from build123d import *

# Parameters (mm, degrees)
CROQUIS2_W                 = 25
CROQUIS2_H                 = 50
SALIENTE_EXTRUIR2_DEPTH    = 20
CROQUIS19_W                = 25
CROQUIS19_H                = 20
SALIENTE_EXTRUIR8_DEPTH    = 6
CORTAR_EXTRUIR1_DEPTH      = 9
CORTAR_EXTRUIR2_DEPTH      = 39.951893407
CORTAR_EXTRUIR2_DEPTH_BACK = 39.951893407
CROQUIS9_R                 = 8
CORTAR_EXTRUIR3_DEPTH      = 5
SALIENTE_EXTRUIR9_DEPTH    = 2
CROQUIS11_W                = 13
CROQUIS11_H                = 2
SALIENTE_EXTRUIR4_DEPTH    = 6
CROQUIS13_W                = 13
CROQUIS13_H                = 2
SALIENTE_EXTRUIR5_DEPTH    = 6
CROQUIS16_R                = 1.75
CORTAR_EXTRUIR6_DEPTH      = 43.793106922
CROQUIS17_W                = 13
CROQUIS17_H                = 8
SALIENTE_EXTRUIR7_DEPTH    = 11
REDONDEO1_R                = 4
CROQUIS12_R                = 1.75
CORTAR_EXTRUIR4_DEPTH      = 46.180194776
CROQUIS14_R                = 1.75
CORTAR_EXTRUIR5_DEPTH      = 46.180194776
CROQUIS18_R                = 1.75
CORTAR_EXTRUIR7_DEPTH      = 48.796443382
REDONDEO1_OF_SIMETR_A1_R   = 4
CROQUIS23_W                = 25
CROQUIS23_H                = 18
CORTAR_EXTRUIR9_DEPTH      = 6
CHAFL_N1_SIZE              = 12


with BuildPart() as part:
    # Croquis2 → Saliente-Extruir2 (new body)
    with BuildSketch(Plane(origin=(0, 0, 0), x_dir=(1, 0, 0), z_dir=(0, 1, 0))):
        Rectangle(CROQUIS2_W, CROQUIS2_H)
    extrude(amount=SALIENTE_EXTRUIR2_DEPTH)

    # Croquis19 → Saliente-Extruir8 (add)
    with BuildSketch(Plane.XY.offset(25)):
        with Locations((0, 10)):
            Rectangle(CROQUIS19_W, CROQUIS19_H)
    extrude(amount=SALIENTE_EXTRUIR8_DEPTH)

    # Croquis4 → Cortar-Extruir1 (cut, symmetric)
    with BuildSketch(Plane(origin=(0, 0, 0), x_dir=(0, 0, -1), z_dir=(1, 0, 0))):
        with BuildLine():
            Line((-26, 4), (-3, 4))
            ThreePointArc((-3, 4), (8.313708499, 8.686291501), (13, 20))
            Line((13, 20), (-26, 20))
            Line((-26, 20), (-26, 4))
        make_face()
    extrude(amount=CORTAR_EXTRUIR1_DEPTH, both=True, mode=Mode.SUBTRACT)

    # Croquis5 → Cortar-Extruir2 (cut, two sides: drawn at the far end of the back side and taken through both)
    with BuildSketch(Plane(origin=(0, 0, 0), x_dir=(0, 0, -1), z_dir=(1, 0, 0)).offset(-CORTAR_EXTRUIR2_DEPTH_BACK)):
        with BuildLine():
            ThreePointArc((2.6, 20), (-3, 25.6), (-8.6, 20))
            Line((-8.6, 20), (2.6, 20))
        make_face()
        with BuildLine():
            Line((2.6, 20), (-8.6, 20))
            ThreePointArc((-8.6, 20), (-3, 14.4), (2.6, 20))
        make_face()
    extrude(amount=CORTAR_EXTRUIR2_DEPTH + CORTAR_EXTRUIR2_DEPTH_BACK, mode=Mode.SUBTRACT)

    # Croquis9 → Cortar-Extruir3 (cut)
    with BuildSketch(Plane.XY.offset(31)):
        with Locations((0, 20)):
            Circle(CROQUIS9_R)
    extrude(amount=-CORTAR_EXTRUIR3_DEPTH, mode=Mode.SUBTRACT)

    # Croquis22 → Saliente-Extruir9 (add)
    with BuildSketch(Plane.XY.offset(31)):
        with BuildLine():
            Line((6, 20), (12.5, 20))
            Line((12.5, 20), (12.5, 0))
            Line((12.5, 0), (-12.5, 0))
            Line((-12.5, 0), (-12.5, 20))
            Line((-12.5, 20), (-6, 20))
            ThreePointArc((-6, 20), (0, 14), (6, 20))
        make_face()
    extrude(amount=SALIENTE_EXTRUIR9_DEPTH)

    # Croquis11 → Saliente-Extruir4 (add)
    with BuildSketch(Plane(origin=(12.5, 0, 0), x_dir=(0, 0, -1), z_dir=(1, 0, 0))):
        with Locations((-26.5, 19)):
            Rectangle(CROQUIS11_W, CROQUIS11_H)
    extrude(amount=SALIENTE_EXTRUIR4_DEPTH)

    # Croquis13 → Saliente-Extruir5 (add)
    with BuildSketch(Plane.ZY.offset(12.5)):
        with Locations((26.5, 19)):
            Rectangle(CROQUIS13_W, CROQUIS13_H)
    extrude(amount=SALIENTE_EXTRUIR5_DEPTH)

    # Croquis16 → Cortar-Extruir6 (cut, through all)
    with BuildSketch(Plane(origin=(0, 20, 0), x_dir=(1, 0, 0), z_dir=(0, 1, 0))):
        with Locations(Location((-7.5, 22, 0), (0, 0, 270))):
            Circle(CROQUIS16_R)
        with Locations(Location((7.5, 22, 0), (0, 0, 270))):
            Circle(CROQUIS16_R)
    extrude(amount=-CORTAR_EXTRUIR6_DEPTH, mode=Mode.SUBTRACT)

    # Croquis17 → Saliente-Extruir7 (add)
    with BuildSketch(Plane.ZY.offset(12.5)):
        with Locations((3, 4)):
            Rectangle(CROQUIS17_W, CROQUIS17_H)
    saliente_extruir7 = extrude(amount=SALIENTE_EXTRUIR7_DEPTH)

    # Redondeo1
    redondeo1_edges = [part.edges().sort_by_distance(p)[0] for p in [
        (-23.5, 0, 3),
        (-23.5, 8, 3),
    ]]
    fillet(redondeo1_edges, radius=REDONDEO1_R - 0.0001)  # a hair under: the kernel refuses the full size

    # Croquis12 → Cortar-Extruir4 (cut, through all)
    with BuildSketch(Plane(origin=(0, 20, 0), x_dir=(1, 0, 0), z_dir=(0, 1, 0))):
        with Locations(Location((15.5, -23, 0), (0, 0, 270))):
            Circle(CROQUIS12_R)
        with Locations(Location((15.5, -30, 0), (0, 0, 270))):
            Circle(CROQUIS12_R)
    extrude(amount=-CORTAR_EXTRUIR4_DEPTH, mode=Mode.SUBTRACT)

    # Croquis14 → Cortar-Extruir5 (cut, through all)
    with BuildSketch(Plane(origin=(0, 20, 0), x_dir=(1, 0, 0), z_dir=(0, 1, 0))):
        with Locations(Location((-15.5, -23, 0), (0, 0, 270))):
            Circle(CROQUIS14_R)
        with Locations(Location((-15.5, -30, 0), (0, 0, 270))):
            Circle(CROQUIS14_R)
    extrude(amount=-CORTAR_EXTRUIR5_DEPTH, mode=Mode.SUBTRACT)

    # Croquis18 → Cortar-Extruir7 (cut, through all)
    with BuildSketch(Plane(origin=(0, 0, -3.5), x_dir=(-1, 0, 0), z_dir=(0, 0, -1))):
        with Locations((19.5, 4)):
            Circle(CROQUIS18_R)
    cortar_extruir7 = extrude(amount=-CORTAR_EXTRUIR7_DEPTH, mode=Mode.SUBTRACT)

    # Simetría1: Saliente-Extruir7, Cortar-Extruir7 across plane
    add(saliente_extruir7.mirror(Plane(origin=(0, 0, 0), x_dir=(0, 0, 1), z_dir=(1, 0, 0))))
    add(cortar_extruir7.mirror(Plane(origin=(0, 0, 0), x_dir=(0, 0, 1), z_dir=(1, 0, 0))), mode=Mode.SUBTRACT)

    # Redondeo1 of Simetría1
    redondeo1_of_simetr_a1_edges = [part.edges().sort_by_distance(p)[0] for p in [
        (23.5, 0, 3),
        (23.5, 8, 3),
    ]]
    fillet(redondeo1_of_simetr_a1_edges, radius=REDONDEO1_OF_SIMETR_A1_R - 0.0001)  # a hair under: the kernel refuses the full size

    # Croquis23 → Cortar-Extruir9 (cut)
    with BuildSketch(Plane(origin=(0, 0, -25), x_dir=(-1, 0, 0), z_dir=(0, 0, -1))):
        with Locations((0, 9)):
            Rectangle(CROQUIS23_W, CROQUIS23_H)
    extrude(amount=-CORTAR_EXTRUIR9_DEPTH, mode=Mode.SUBTRACT)

    # Chaflán1
    chafl_n1_edges = [part.edges().sort_by_distance(p)[0] for p in [
        (0, 0, -19),
    ]]
    chamfer(chafl_n1_edges, length=CHAFL_N1_SIZE)


solid = part.part
Input: part model. Units: mm. Frame: model coordinates. A direction names the side the tool comes from. Coordinates: 2 decimals unless noted, no trailing zeros. Loops run counter-clockwise (first coordinate to the right, second up) from the corner with the lowest first, then second, coordinate; pieces in that order, holes last. Notation, with made-up numbers: (-20.5, 8) -> (10.5, 8) arc R24 cw to (10.5, 25) -> close; hole circle Ø9 at (15, 80). An arc over 180 degrees is marked (long way). Write item = value, one per line. Start each with the question number.
Item 1: Cut plane C-C, the plane y = 9.5. Return loops of the section in (x, z).
Item 2: First-contact query: P1, Ø12, axis at y = 13, z = -18.5, coming from the -X side; P2, Ø1, axis at x = -14.5, y = 18.5, coming from the -Z side; P3, Ø9, axis at x = -20.5, y = 3.5, coming from the -Z side; P4, Ø3, axis at x = 19.5, y = 4, coming from the +Z side. Flat tips, straight axial feed; report the tip coordinate or a pass-through.
Item 3: Material intervals for line 1 (X direction, y = 19.45, z = -22); line 2 (X direction, y = 18.5, z = 23); line 3 (X direction, y = 5, z = -1.5), sorted ascending.
Item 4: Cut plane A-A, the plane z = 23. Return loops of the section in (x, y), plus the area to 3 significant figures.
Item 5: Cut plane D-D, the plane z = 30. Return loops of the section in (x, y).
Item 6: Mould query, pull axis Y, two halves, no side actions, for faces 4 (the face through (-17, 4, 9.5)), 5 (the face through (0, 18, -22)), 6 (the face through (-18.11, 2.94, 2.91)). Classes: pulls with the +Y half, pulls with the -Y half, needs draft (parallel to the pull), parting line crosses it, or undercut.
Item 7: Cut plane B-B, the plane x = 15.5. Return loops of the section in (y, z), plus the area to 3 significant figures.
Item 8: Reachability of faces 1 (the face through (0, 12, 29)), 2 (the face through (0, 14, 32)), 3 (the face through (-15, 19, 20)) from +Z, -Z, +X, -X, +Y, -Y: full face, straight path, thin tool, end or side. Return the list, or none.
Ans:
q1.outline = (-12.5, -16.5) -> (12.5, -16.5) -> (12.5, 33) -> (-12.5, 33) -> close; hole (-9, -9.07) -> (9, -9.07) -> (9, 26) -> (-9, 26) -> close
q2.P1 = -12.5
q2.P2 = 20
q2.P3 = -3.5
q2.P4 = through
q3.line_1 = -12.5 to -9.25, -5.75 to 5.75, 9.25 to 12.5
q3.line_2 = -18.5 to -17.25, -13.75 to -9, 9 to 13.75, 17.25 to 18.5
q3.line_3 = -23.37 to -20.94, -18.06 to -9, 9 to 18.06, 20.94 to 23.37
q4.outline = (-18.5, 18) -> (-17.25, 18) -> (-17.25, 20) -> (-18.5, 20) -> close; (-13.75, 18) -> (-12.5, 18) -> (-12.5, 0) -> (12.5, 0) -> (12.5, 18) -> (13.75, 18) -> (13.75, 20) -> (9, 20) -> (9, 4) -> (-9, 4) -> (-9, 20) -> (-13.75, 20) -> close; (17.25, 18) -> (18.5, 18) -> (18.5, 20) -> (17.25, 20) -> close
q4.area = 222 mm²
q5.outline = (-18.5, 18) -> (-17.25, 18) -> (-17.25, 20) -> (-18.5, 20) -> close; (-13.75, 18) -> (-12.5, 18) -> (-12.5, 0) -> (12.5, 0) -> (12.5, 18) -> (13.75, 18) -> (13.75, 20) -> (8, 20) arc R8 cw to (-8, 20) -> (-13.75, 20) -> close; (17.25, 18) -> (18.5, 18) -> (18.5, 20) -> (17.25, 20) -> close
q6.face_4 = needs draft
q6.face_5 = pulls with the -Y half
q6.face_6 = undercut
q7.outline = (0, -3.5) -> (8, -3.5) -> (8, 9.5) -> (0, 9.5) -> close; (18, 20) -> (20, 20) -> (20, 21.25) -> (18, 21.25) -> close; (18, 24.75) -> (20, 24.75) -> (20, 28.25) -> (18, 28.25) -> close; (18, 31.75) -> (20, 31.75) -> (20, 33) -> (18, 33) -> close
q7.area = 116 mm²
q8.face_1 = +Y
q8.face_2 = +Z, +Y
q8.face_3 = -Z, -X, +Y, -Y
